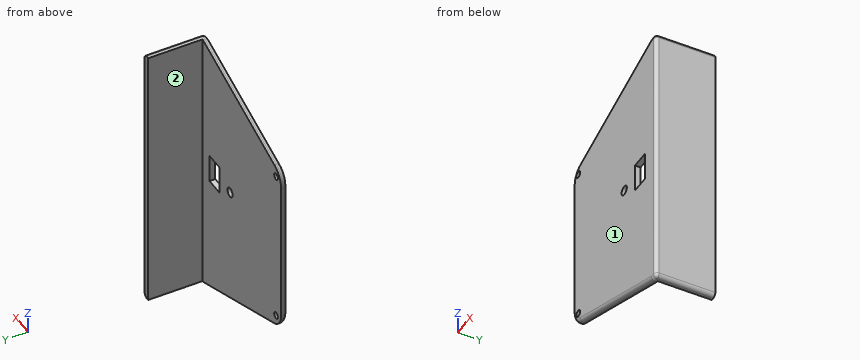
from build123d import *

# Parameters (mm, degrees)
BOSS_EXTRUDE1_DEPTH     = 3
SKETCH2_W               = 3.3999999999999995
SKETCH2_H               = 144.72
BOSS_EXTRUDE2_DEPTH     = 31.5
SKETCH3_R               = 1.749999999999997
CUT_EXTRUDE1_DEPTH      = 40
FILLET1_R               = 2
FILLET2_R               = 2
CONG_1_R                = 10
ESQUISSE2_R             = 2.500000000000002
ENL_V_MAT_EXTRU_1_DEPTH = 10


with BuildPart() as part:
    # Sketch1 → Boss-Extrude1 (new body)
    with BuildSketch(Plane(origin=(0, 0, 0), x_dir=(1, 0, 0), z_dir=(0, 1, 0))):
        Polygon((-79.17599616899001, 45), (-79.17599616899001, -45), (-4, -72.36), (0, -72.36), (0, 72.36), (-4, 72.36), align=None)
    extrude(amount=BOSS_EXTRUDE1_DEPTH)

    # Sketch2 → Boss-Extrude2 (add)
    with BuildSketch(Plane.XZ):
        with Locations((-1.6999999999999997, 0)):
            Rectangle(SKETCH2_W, SKETCH2_H)
    extrude(amount=-BOSS_EXTRUDE2_DEPTH)

    # Sketch3 → Cut-Extrude1 (cut)
    with BuildSketch(Plane(origin=(0, 3, 0), x_dir=(1, 0, 0), z_dir=(0, 1, 0))):
        with Locations(Location((-74.2610839032561, -41.5585413818937, 0), (0, 0, 270))):
            Circle(SKETCH3_R)
        with Locations(Location((-74.26108390325611, 41.55854138189368, 0), (0, 0, 270))):
            Circle(SKETCH3_R)
    extrude(amount=-CUT_EXTRUDE1_DEPTH, mode=Mode.SUBTRACT)

    # Fillet1
    fillet1_edges = [part.edges().sort_by_distance(p)[0] for p in [
        (-2, 0, -72.36),
        (0, 0, 0),
        (-2, 0, 72.36),
        (-41.587998084495005, 0, 58.68),
        (-79.17599616899001, 0, 0),
        (-41.587998084495005, 0, -58.68),
    ]]
    fillet(fillet1_edges, radius=FILLET1_R)

    # Fillet2
    # the kernel refuses this fillet: 2 mm, written as the material it takes off along each edge
    with BuildSketch(Plane(origin=(-2, 2, -70.36), x_dir=(1, 0, 0), z_dir=(0, 0, -1))) as fillet2_piece_1_section:
        Polygon((0, 0), (FILLET2_R, 0), (FILLET2_R, FILLET2_R), (0, FILLET2_R), align=None)
    fillet2_piece_1 = extrude(amount=FILLET2_R, mode=Mode.PRIVATE)
    fillet2_piece_1 = fillet2_piece_1 - Plane(origin=(-2, 2, -70.36), x_dir=(-0.7071067811865475, 0.7071067811865475, 0), z_dir=(0, 0, -1)) * Sphere(FILLET2_R, mode=Mode.PRIVATE)
    add(fillet2_piece_1, mode=Mode.SUBTRACT)
    with BuildSketch(Plane(origin=(-2, 2, 70.36), x_dir=(1, 0, 0), z_dir=(0, 0, 1))) as fillet2_piece_2_section:
        Polygon((0, 0), (FILLET2_R, 0), (FILLET2_R, -FILLET2_R), (0, -FILLET2_R), align=None)
    fillet2_piece_2 = extrude(amount=FILLET2_R, mode=Mode.PRIVATE)
    fillet2_piece_2 = fillet2_piece_2 - Plane(origin=(-2, 2, 70.36), x_dir=(-0.7071067811865475, 0.7071067811865475, 0), z_dir=(0, 0, 1)) * Sphere(FILLET2_R, mode=Mode.PRIVATE)
    add(fillet2_piece_2, mode=Mode.SUBTRACT)
    with BuildSketch(Plane(origin=(0, 36.5, -72.36), x_dir=(-1, 0, 0), z_dir=(0, -1, 0))) as fillet2_piece_3:
        with BuildLine():
            CenterArc((FILLET2_R, -FILLET2_R), FILLET2_R, 90, 90)
            Line((-2.2e-16, -FILLET2_R), (0, 0))
            Line((0, 0), (FILLET2_R, 0))
        make_face()
    extrude(amount=34.5, mode=Mode.SUBTRACT)
    with BuildSketch(Plane(origin=(0, 1.9999999999999993, 72.36), x_dir=(-1, 0, 0), z_dir=(0, 1, 0))) as fillet2_piece_4:
        with BuildLine():
            CenterArc((FILLET2_R, -FILLET2_R), FILLET2_R, 90, 90)
            Line((0, -FILLET2_R), (0, 0))
            Line((0, 0), (FILLET2_R, 0))
        make_face()
    extrude(amount=34.5, mode=Mode.SUBTRACT)

    # Congé1
    # the kernel refuses this fillet: 10 mm, written as the material it takes off along each edge
    with BuildSketch(Plane(origin=(-69.17599616899001, 0, -37.99776488738916), x_dir=(-1, 0, 0), z_dir=(0, 0, 1))) as cong_1_piece_1:
        with BuildLine():
            CenterArc((8, -2), 2, 0, 90)
            Line((10, -2), (10, 0))
            Line((10, 0), (8, 0))
        make_face()
    revolve(axis=Axis((-69.17599616899001, 0, -37.99776488738916), (0, -1, 0)), revolution_arc=70.00122819209012, mode=Mode.SUBTRACT)
    with BuildSketch(Plane(origin=(-69.17599616899001, 0, 37.99776488738917), x_dir=(-0.34199999999999997, 0, 0.9396999521123751), z_dir=(0.9396999521123751, 0, 0.34199999999999997))) as cong_1_piece_2:
        with BuildLine():
            CenterArc((8, -2), 2, 0, 90)
            Line((10, -2), (10, 0))
            Line((10, 0), (8, 0))
        make_face()
    revolve(axis=Axis((-69.17599616899001, 0, 37.99776488738917), (0, -1, 0)), revolution_arc=70.00122819209012, mode=Mode.SUBTRACT)
    with BuildSketch(Plane(origin=(-79.17599616899001, -4.4e-16, 45), x_dir=(0, 0, -1), z_dir=(0, 1, 0))) as cong_1_piece_3:
        with BuildLine():
            CenterArc((CONG_1_R * 0.700223511261, -CONG_1_R), CONG_1_R, 90, 70.00122819209011)
            Line((-CONG_1_R * 0.239476440851, -CONG_1_R * 0.658), (0, 0))
            Line((0, 0), (CONG_1_R * 0.700223511261, 0))
        make_face()
    extrude(amount=20.505587781527105, mode=Mode.SUBTRACT)
    with BuildSketch(Plane(origin=(-79.17599616899001, -4.4e-16, -45), x_dir=(0, 0, 1), z_dir=(0, 1, 0))) as cong_1_piece_4:
        with BuildLine():
            CenterArc((CONG_1_R * 0.700223511261, CONG_1_R), CONG_1_R, 199.99877180790997, 70.00122819209003)
            Line((-CONG_1_R * 0.239476440851, CONG_1_R * 0.658), (0, 0))
            Line((0, 0), (CONG_1_R * 0.700223511261, 0))
        make_face()
    extrude(amount=20.5055877815271, mode=Mode.SUBTRACT)

    # Esquisse2 → Enlèv. mat.-Extru.1 (cut)
    with BuildSketch(Plane.XZ):
        with Locations(Location((-30, -3.67e-15, 0), (0, 0, 270))):
            Circle(ESQUISSE2_R)
        Polygon((-10.25, 7.499999999999999), (-19.75, 7.499999999999999), (-19.749999999999996, -7.500000000000002), (-10.249999999999998, -7.500000000000001), align=None)
    extrude(amount=-ENL_V_MAT_EXTRU_1_DEPTH, mode=Mode.SUBTRACT)


solid = part.part
Verification items for the finished model (mm, model axes). Face numbers are marked on the shaded views. A direction names the side the tool comes from. Give positions to 0.01 mm unless a question says otherwise; leave off trailing zeros. Write each loop counter-clockwise with the first axis right and the second up, starting at its lowest first coordinate (ties: lowest second). Pieces come first, ordered by that corner, then holes.
(1) Cross-section at C-C (y = 17.5). Enter the section's corners in (x, z), plus the area to 3 significant figures.
(2) Cross-section at A-A (z = 0). Enter the section's corners in (x, y).
(3) Gauge pin test, flat ends, axial feed: pin 1 (1 mm diameter, centred on y = 16, z = -34.5, fed in from -X); pin 2 (0.9 mm diameter, centred on y = 1.5, z = 2, fed in from +X); pin 3 (6 mm diameter, centred on x = -30, z = 0, fed in from +Y); pin 4 (1.5 mm diameter, centred on x = -14.5, y = 1.5, fed in from +Z). Record the tip position at first contact, or that the pin passes through.
(4) Cross-section at B-B (z = -18). Enter the section's corners in (x, y), plus the area to 3 significant figures.
(5) Material ranges on line 1 (X direction, y = 1.9, z = 0); line 2 (X direction, y = 17, z = 6); line 3 (X direction, y = 1, z = 0), recorded low to high.
(6) Access from +Z, -Z, +X, -X, +Y, -Y to the whole of each face (thin tool, end or side, straight path). Record for the marked faces 1 and 2.
Worked out:
1. outline: (-3.4, -72.36) - (-2, -72.36) arc R2 ccw to (0, -70.36) - (0, 70.36) arc R2 ccw to (-2, 72.36) - (-3.4, 72.36) - close
1. area: 490 mm2
2. outline: (-79.18, 2) arc R2 ccw to (-77.18, 0) - (-32.5, 0) - (-32.5, 3) - (-79.18, 3) - close; (-27.5, 0) - (-19.75, 0) - (-19.75, 3) - (-27.5, 3) - close; (-10.25, 0) - (-2, 0) arc R2 ccw to (0, 2) - (0, 31.5) - (-3.4, 31.5) - (-3.4, 3) - (-10.25, 3) - close
3. pin 1: stops at x = -3.4
3. pin 2: stops at x = 0
3. pin 3: stops at y = 3
3. pin 4: stops at z = 68.78
4. outline: (-79.18, 2) arc R2 ccw to (-77.18, 0) - (-2, 0) arc R2 ccw to (0, 2) - (0, 31.5) - (-3.4, 31.5) - (-3.4, 3) - (-79.18, 3) - close
4. area: 333 mm2
5. line 1: x = -79.17 to -32.5, -27.5 to -19.75, -10.25 to 0
5. line 2: x = -3.4 to 0
5. line 3: x = -78.91 to -32.5, -27.5 to -19.75, -10.25 to -0.27
6. face 1: +Z, -Z, +X, -X, -Y
6. face 2: +Z, -Z, -X, +Y
